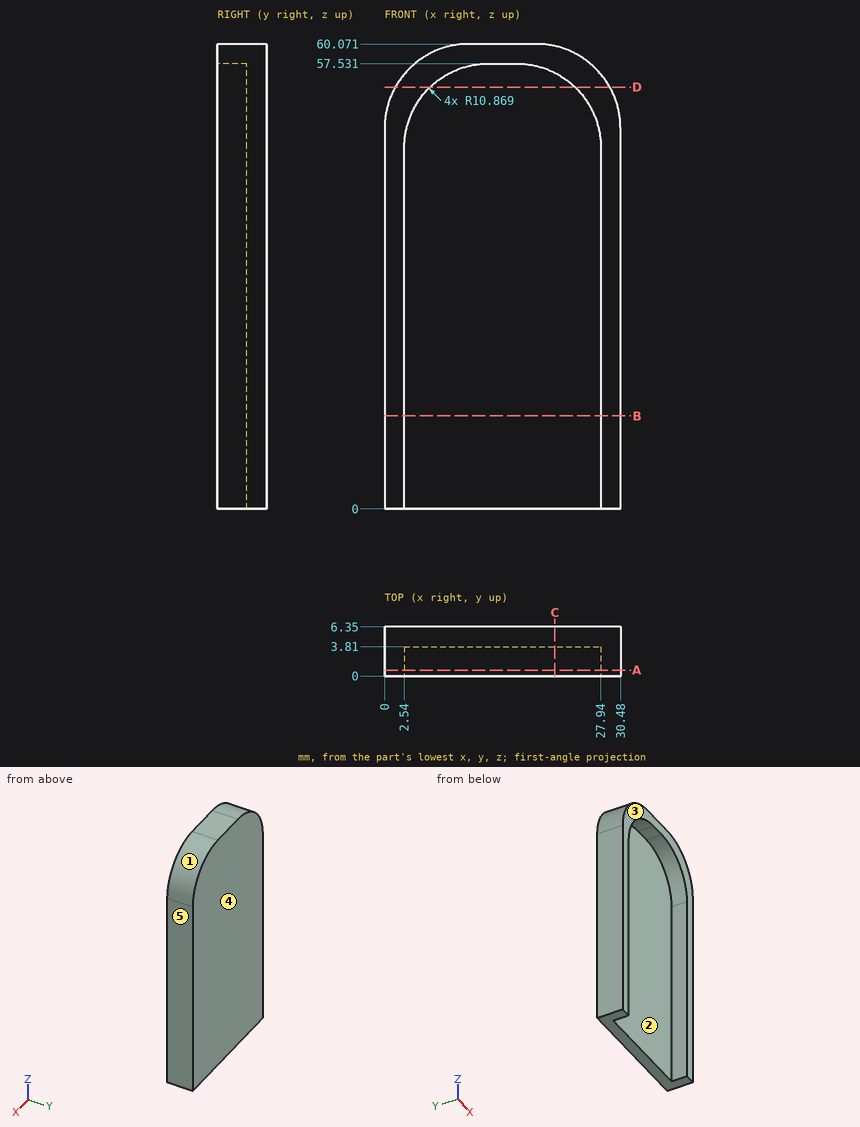
For this review, use the dimensioned drawing (mm, ordinates from the lowest corner) and the shaded views. A direction names the side the tool comes from. Give positions to 0.01 mm unless a question says otherwise; leave off trailing zeros. Write each loop counter-clockwise with the first axis right and the second up, starting at its lowest first coordinate (ties: lowest second). Pieces come first, ordered by that corner, then holes. Notation, with made-up numbers: M 36,-6.5 L 81,-6.5 A38 cw 81,31.5 Z; hole C 72.25,4 d6. An arc over 180 degrees is marked long. Answer as a JSON object with one key per item and string values. Group by question number.
Item 1: Consider section A-A on y = 0.75. Write out the cut boundary in (x, z).
Item 2: Draft analysis for pull direction Y (two halves, no side actions). For the marked faces 3, 4 and 5, state which applies: +Y half, -Y half, draft (parallel to the pull), parting line (faces both ways), or undercut.
Item 3: For probe 1 along X at (y, z) = (3.25, 37); probe 2 along Y at (x, z) = (7, 45); probe 3 along Z at (x, y) = (14, 3.5), list the stretches that pass through material, from the lowest coordinate up. Write a range as [from, to].
Item 4: Consider section C-C on x = 22. Write out the cut boundary in (y, z) (3 decimals).
Item 5: Tool access review of the marked faces 1 and 2: name each direction out of +Z, -Z, +X, -X, +Y, -Y from which nothing blocks a thin tool from reaching the whole face with its end or side.
Item 6: Consider section B-B on z = 12. Write out the cut boundary in (x, y).
Item 7: For pin 1 Ø5 at (x, z) = (14.5, 41) entering from -Y; pin 2 Ø3 at (x, y) = (16, 1.5) entering from -Z, all flat-tipped, find the tip position at first contact; note any pin that passes through.
Item 8: Consider section D-D on z = 54.5. Write out the cut boundary in (x, y).
Check result:
{
 "1": {"outline": "M 0,0 L 2.54,0 L 2.54,46.66 A10.87 cw 13.41,57.53 L 17.07,57.53 A10.87 cw 27.94,46.66 L 27.94,0 L 30.48,0 L 30.48,49.2 A10.87 ccw 19.61,60.07 L 10.87,60.07 A10.87 ccw 0,49.2 Z"},
 "2": {"face 3": "-Y half", "face 4": "+Y half", "face 5": "draft"},
 "3": {"probe 1": "x = [0, 2.54], [27.94, 30.48]", "probe 2": "y = [3.81, 6.35]", "probe 3": "z = [57.53, 60.07]"},
 "4": {"outline": "M 0,56.349 L 3.81,56.349 L 3.81,0 L 6.35,0 L 6.35,59.805 L 0,59.805 Z"},
 "5": {"face 1": "+Z, +X, +Y, -Y", "face 2": "-Z, -Y"},
 "6": {"outline": "M 0,0 L 2.54,0 L 2.54,3.81 L 27.94,3.81 L 27.94,0 L 30.48,0 L 30.48,6.35 L 0,6.35 Z"},
 "7": {"pin 1": "stops at y = 3.81", "pin 2": "stops at z = 57.52"},
 "8": {"outline": "M 1.38,0 L 5.88,0 L 5.88,3.81 L 24.6,3.81 L 24.6,0 L 29.1,0 L 29.1,6.35 L 1.38,6.35 Z"}
}
